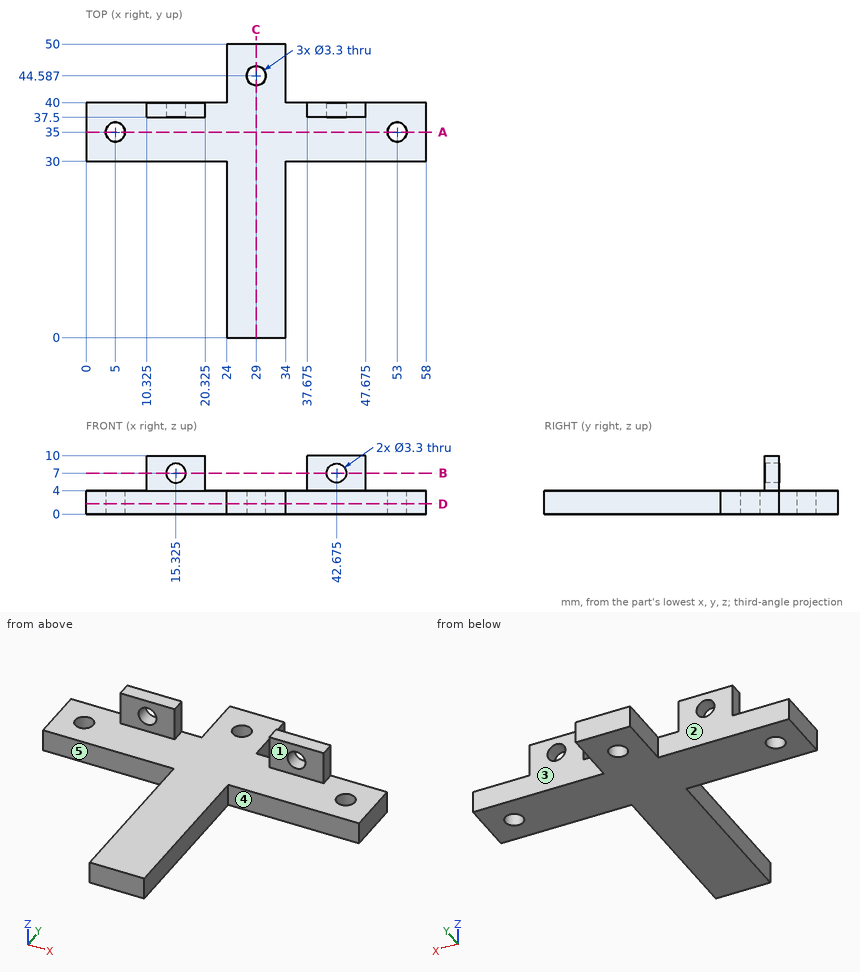
Could you check a few things on this drawing? It's one solid part, dimensions in mm from its lowest x, y, z. A direction names the side the tool comes from. Give positions to 0.01 mm unless a question says otherwise; leave off trailing zeros. Order: outer loops, then holes, each group sorted by start corner. A loop starts at its lowest first (then second) coordinate and runs counter-clockwise, first axis right, second up. Notation, with made-up numbers: (10.5, -32.5) - (25.5, -32.5) arc R17 ccw to (25.5, -22.5) - close; hole circle Ø9 at (1.25, -12). An arc over 180 degrees is marked (long way). Return JSON: item names as keys, results as strings. Group by question number.
Q1. Please list where these lines run through material, in increasing order: line 1 along Y through (x, z) = (29, 1.75); line 2 along Y through (x, z) = (5, 3.2); line 3 along X through (y, z) = (39, 9) (1 decimal). Write a range as [from, to].
Q2. Suppose I cut it at B-B, the plane z = 7. Please give me the cut outline in (x, y) (1 decimal).
Q3. Suppose I cut it at D-D, the plane z = 1.75. Please give me the cut outline in (x, y).
Q4. Which directions (+Z, -Z, +X, -X, +Y, -Y) give clear straight access to the entire face, cutting with the end or side of a thin tool? Please do the marked faces 1, 2, 3, 4 and 5.
Q5. Suppose I cut it at C-C, the plane x = 29. Please give me the cut outline in (y, z), and give its area (3 significant figures).
Q6. Suppose I cut it at A-A, the plane y = 35. Please give me the cut outline in (x, z).
Q7. Will these pins go through, and if not, where does the flat tip stop? pin 1 Ø5 at (y, z) = (10.5, 4) entering from +X; pin 2 Ø5 at (x, z) = (40, 5) entering from +Y; pin 3 Ø5.5 at (x, y) = (5, 35) entering from +Z.
Resolved:
{
 "1": {"line 1": "y = [0, 42.94], [46.24, 50]", "line 2": "y = [30, 33.35], [36.65, 40]", "line 3": "x = [10.3, 20.3], [37.7, 47.7]"},
 "2": {"outline": "(10.3, 37.5) - (13.7, 37.5) - (13.7, 40) - (10.3, 40) - close; (17, 37.5) - (20.3, 37.5) - (20.3, 40) - (17, 40) - close; (37.7, 37.5) - (41, 37.5) - (41, 40) - (37.7, 40) - close; (44.3, 37.5) - (47.7, 37.5) - (47.7, 40) - (44.3, 40) - close"},
 "3": {"outline": "(0, 30) - (24, 30) - (24, 0) - (34, 0) - (34, 30) - (58, 30) - (58, 40) - (34, 40) - (34, 50) - (24, 50) - (24, 40) - (0, 40) - close; hole circle Ø3.3 at (5, 35); hole circle Ø3.3 at (29, 44.59); hole circle Ø3.3 at (53, 35)"},
 "4": {"face 1": "+Z, +X, -X, -Y", "face 2": "+Z, -Z, -X, +Y", "face 3": "+Z, -Z, +X, +Y", "face 4": "+Z, -Z, +X, -Y", "face 5": "+Z, -Z, -X, -Y"},
 "5": {"outline": "(0, 0) - (42.94, 0) - (42.94, 4) - (0, 4) - close; (46.24, 0) - (50, 0) - (50, 4) - (46.24, 4) - close", "area": "187 mm2"},
 "6": {"outline": "(0, 0) - (3.35, 0) - (3.35, 4) - (0, 4) - close; (6.65, 0) - (51.35, 0) - (51.35, 4) - (6.65, 4) - close; (54.65, 0) - (58, 0) - (58, 4) - (54.65, 4) - close"},
 "7": {"pin 1": "stops at x = 34", "pin 2": "stops at y = 40", "pin 3": "stops at z = 4"}
}
